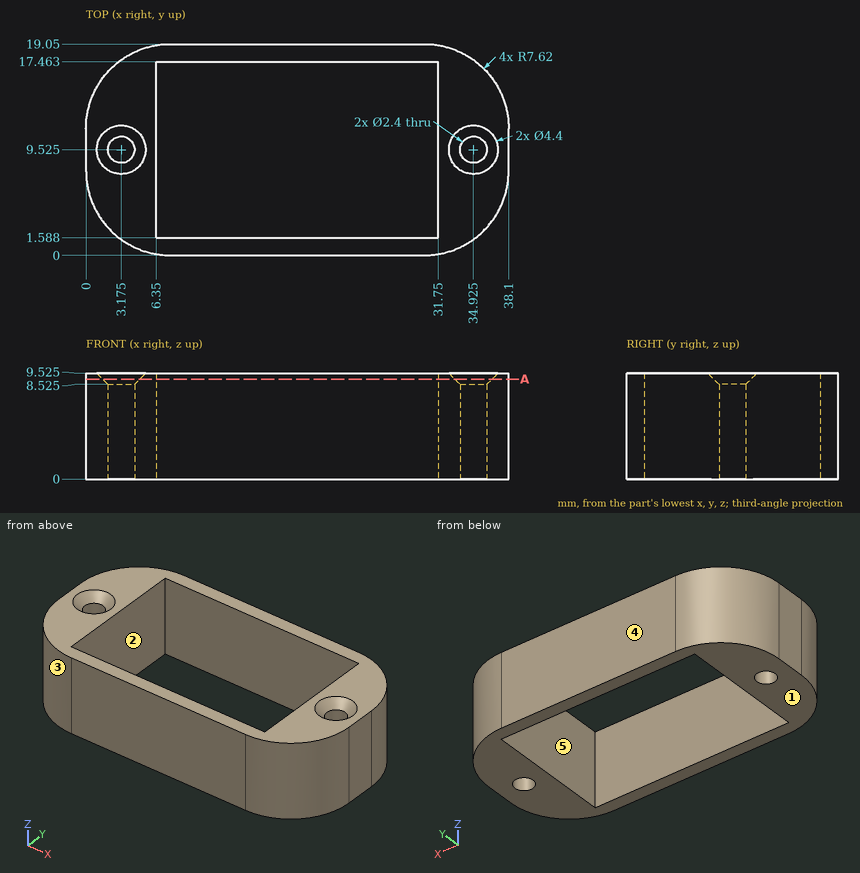
Part print with two shaded views. Sizes in mm from the minimum x, y, z corner. A direction names the side the tool comes from. Round coordinates to 2 decimals unless told otherwise and drop trailing zeros. Put each result on its own line as item: value. Start each with the question number.
Item 1: 3-axis set-ups, long thin cutter, end or side, ignore diameter. For the marked faces 1 and 2: which of +Z, -Z, +X, -X, +Y, -Y reach the whole face in a straight line?
Item 2: Mould opens along X. For the marked faces 3, 4 and 5 say: released by +X, released by -X, zero draft, split by the parting line, or undercut.
Item 3: Drop flat-ended pins along their axis: P1, Ø1.5, axis at x = 30, y = 11, coming from the +Z side; P2, Ø4, axis at x = 34.925, y = 9.525, coming from the +Z side (1 decimal); P3, Ø4, axis at y = 4.5, z = 7, coming from the -X side. Give the stop position or say it passes through.
Item 4: Cut at A-A (z = 9). Give the number of separate pieces and of enclosed holes in the cut face, then the cut area to 3 significant figures.
Item 5: Drill centre lines: line 1 along Y through (x, z) = (23, 5.75); line 2 along X through (y, z) = (8, 7.5); line 3 along X through (y, z) = (5.25, 6.75). Where is each one in solid material? Low to high.
Answer block:
1. face 1: -Z, +X, -X, +Y, -Y
1. face 2: +Z, -Z
2. face 3: released by -X
2. face 4: zero draft
2. face 5: undercut
3. P1: through
3. P2: z = 9.3
3. P3: x = 0.08
4. separate pieces: 1
4. enclosed holes: 3
4. area: 255 mm2
5. line 1: 0 to 1.59, 17.46 to 19.05
5. line 2: 0 to 6.35, 31.75 to 38.1
5. line 3: 0.38 to 6.35, 31.75 to 37.72
